Autodesk Inventor part; units mm, degrees
ref_plane "YZ Plane" through (0, 0, 0) normal (1, 0, 0) x (0, 1, 0)
ref_plane "XZ Plane" through (0, 0, 0) normal (0, 1, 0) x (-1, 0, 0)
ref_plane "XY Plane" through (0, 0, 0) normal (0, 0, 1) x (1, 0, 0)
sketch "Sketch1" plane through (0, 0, 0) normal (0, 0, 1) x (1, 0, 0)
  line L0 (-175, -7.5) -> (-230, -7.5)
  line L1 (-250, 2.5) -> (-152.5, 2.5)
  line L2 (-82.5, -57.5) -> (-255, -57.5)
  line L3 (-150, -42.5) -> (-165, -42.5)
  line L4 (-150, 0) -> (-150, -42.5)
  line L5 (-175, -7.5) -> (-165, -17.5)
  line L6 (-165, -42.5) -> (-165, -17.5)
  line L7 (-175, -107.5) -> (-230, -107.5)
  line L8 (-250, -117.5) -> (-152.5, -117.5)
  line L9 (-150, -72.5) -> (-165, -72.5)
  line L10 (-150, -115) -> (-150, -72.5)
  line L11 (-175, -107.5) -> (-165, -97.5)
  line L12 (-165, -72.5) -> (-165, -97.5)
  line L13 (-230, -7.5) -> (-230, -107.5)
  line L14 (-260, -107.5) -> (-260, -7.5)
  line L15 (-250, 2.5) -> (-260, -7.5)
  line L16 (-250, -117.5) -> (-260, -107.5)
  line L17 (-152.5, 2.5) -> (-150, 0)
  line L18 (-152.5, -117.5) -> (-150, -115)
  point P0 (0, 0)
  point P1 (-260, 2.5)
  point P2 (-152.5, 2.5)
  point P3 (-260, -117.5)
  point P4 (-150, 2.5)
  point P5 (-150, -117.5)
  dimension "d2" = -7.5
  dimension "d4" = 10
  dimension "d40" = 15
  dimension "d53" = 10
  dimension "d54" = 10
  dimension "d56" = 65
  dimension "d57" = 30
  dimension "d58" = 10
  dimension "d59" = 10
  dimension "d60" = 10
  dimension "d61" = 10
  dimension "d69" = 45
  dimension "d70" = 2.5
  dimension "d71" = 2.5
  dimension "d72" = 2.5
  dimension "d73" = 2.5
extrude "Extrusion1" add sketch "Sketch1" along normal blind 5
sketch "Sketch3" plane through (0, 0, 5) normal (0, 0, 1) x (1, 0, 0)
  line L0 (-155, 3.7259) -> (-155, -113.632) construction
  line L1 (-150, -42.5) -> (-150, 0) construction
  line L2 (-225, -107.5) -> (-225, -7.5) construction
  line L3 (-225, -57.375) -> (-3.3098, -57.375) construction
  point P0 (0, 0)
  point P1 (-150, 5)
  point P2 (-155, -7.375)
  point P3 (-155, -22.375)
  point P4 (-155, -92.375)
  point P5 (-155, -107.375)
  point P6 (-230, -7.5)
  dimension "d41" = 5
  dimension "d42" = 15
  dimension "d43" = 70
hole "Hole2" at (-155, -7.375, 5) at (-155, -22.375, 5) at (-155, -92.375, 5) at (-155, -107.375, 5) direction (0, 0, -1) diameter 5 end through all
sketch "Sketch4" plane through (0, 0, 5) normal (0, 0, 1) x (1, 0, 0)
  circle A0 centre (-250, -7.5) radius 2.5
  circle A1 centre (-250, -107.5) radius 2.5
  circle A2 centre (-167.5, -5) radius 2.5
  circle A3 centre (-167.5, -110) radius 2.5
  point P0 (0, 0)
hole "Hole3" at (-167.5, -5, 5) at (-167.5, -110, 5) at (-250, -107.5, 5) at (-250, -7.5, 5) direction (0, 0, -1) diameter 5 end through all
properties part number "MarcoV2" material "MDF Medium Density Fiberboard"
CAD build for the part. Positions are in the model's coordinates, mm. A direction names the side the tool comes from. Coordinates: 2 decimals unless noted, no trailing zeros. Order: outer loops, then holes, each group sorted by start corner. A loop starts at its lowest first (then second) coordinate and runs counter-clockwise, first axis right, second up. Notation, with made-up numbers: (39.5, 35.5) -> (89.5, 35.5) arc R33 cw to (89.5, 69.5) -> close; hole circle Ø1 at (65.25, -23.5). An arc over 180 degrees is marked (long way). Use one line per item in the form item = value. Start each with the question number.
1) Band-saw the part on C-C on z = 1.25. State how many separate pieces and enclosed holes the cut face has, then the cut area to 3 significant figures.
2) Band-saw the part on A-A on x = -211. Give the cut face in (y, z), then the cut area to 3 significant figures.
3) Band-saw the part on D-D on y = -58. Give the cut face in (x, z).
4) Band-saw the part on B-B on y = -36. Give the cut face in (x, z).
5) Drill centre lines: L1, parallel to Y at x = -155, z = 3.5 (3 decimals); L2, parallel to X at y = -96.5, z = 4; L3, parallel to X at y = -24, z = 3.7. Where is each one in solid material? Low to high. Write a range as [from, to].
6) Pull direction X, two halves, no side cores. Call faces 1 (the flat face through (-150, -21, 2)), 2 (the flat face through (-254.9, -2.4, 2.5)), 3 (the cylindrical face through (-252.48, -7.17, 2.46)): +X half, -X half, draft (parallel to the pull), parting line (faces both ways), or undercut.
7) Tool access for faces 4 (the flat face through (-202, -107.5, 2)), 5 (the flat face through (-230.2, -56.7, 5)): list every direction of +Z, -Z, +X, -X, +Y, -Y with a clear straight run to the whole face (end or side of a thin tool).
Entries:
q1.separate_pieces = 1
q1.enclosed_holes = 8
q1.area = 6,090 mm2
q2.outline = (-117.5, 0) -> (-107.5, 0) -> (-107.5, 5) -> (-117.5, 5) -> close; (-7.5, 0) -> (2.5, 0) -> (2.5, 5) -> (-7.5, 5) -> close
q2.area = 100 mm2
q3.outline = (-260, 0) -> (-230, 0) -> (-230, 5) -> (-260, 5) -> close
q4.outline = (-260, 0) -> (-230, 0) -> (-230, 5) -> (-260, 5) -> close; (-165, 0) -> (-150, 0) -> (-150, 5) -> (-165, 5) -> close
q5.L1 = [-117.5, -109.875], [-104.875, -94.875], [-89.875, -72.5], [-42.5, -24.875], [-19.875, -9.875], [-4.875, 2.5]
q5.L2 = [-260, -230], [-165, -150]
q5.L3 = [-260, -230], [-165, -156.9], [-153.1, -150]
q6.face_1 = +X half
q6.face_2 = -X half
q6.face_3 = undercut
q7.face_4 = +Z, -Z
q7.face_5 = +Z, +X, -X, +Y, -Y
